Here's how the part is built. I have some questions about the finished solid (model axes, mm). A direction names the side the tool comes from. Round coordinates to 2 decimals unless told otherwise and drop trailing zeros. Loops run counter-clockwise (first coordinate to the right, second up) from the corner with the lowest first, then second, coordinate; pieces in that order, holes last. Notation, with made-up numbers: (-12.5, -33) - (4.5, -33) arc R16 ccw to (4.5, -14) - close; hole circle Ø11 at (-29, 0.25). An arc over 180 degrees is marked (long way). Answer as a JSON object with one key per item and string values. Group by question number.
1) If I drill on line 1 along Z through (x, y) = (0, -3.2); line 2 along Z through (x, y) = (0, -1.25), over which ranges is the centre line in solid material (lowest first)? Write a range as [from, to].
2) Will these pins go through, and if not, where does the flat tip stop? P1, Ø3, axis at y = 2.5, z = 7.5, coming from the -X side; P2, Ø2, axis at x = 4.5, y = 2.5, coming from the +Z side.
3) I want a section at C-C, the plane y = -1.25. Please give me the cut outline in (x, z), then the cut area to 3 significant figures.
4) I want a section at B-B, the plane x = -15. Please give me the cut outline in (y, z), then the cut area to 3 significant figures.
5) Which directions (+Z, -Z, +X, -X, +Y, -Y) give clear straight access to the entire face, cutting with the end or side of a thin tool? Please do faces 1 (the face through (20.03, 3.01, -6.31)), 2 (the face through (-14, -3.5, -21)), 3 (the face through (-5.7, -2.5, -20.5)).
6) I want a section at A-A, the plane z = 0. Please give me the cut outline in (x, y), then the cut area to 3 significant figures.
7) If we mould it in two halves opening along Z, with no side actions, what happens to faces 4 (the face through (-20.633, 0.049, 15.821)), 5 (the face through (-4.336, -0.049, 19.524)), 6 (the face through (-14, 3.5, -21))? For each: pulls with the +Z half, pulls with the -Z half, needs draft (parallel to the pull), parting line crosses it, or undercut.
from build123d import *

# Parameters (mm, degrees)
CROQUIS1_R              = 26
CROQUIS1_R_2            = 20
SALIENTE_EXTRUIR1_DEPTH = 3.5
CROQUIS2_R              = 25
CROQUIS2_R_2            = 21
CORTAR_EXTRUIR1_DEPTH   = 1


with BuildPart() as part:
    # Croquis1 → Saliente-Extruir1 (new body, symmetric)
    with BuildSketch(Plane(origin=(0, 0, 0), x_dir=(1, 0, 0), z_dir=(0, 1, 0))):
        Circle(CROQUIS1_R)
        Circle(CROQUIS1_R_2, mode=Mode.SUBTRACT)
    extrude(amount=SALIENTE_EXTRUIR1_DEPTH, both=True)

    # Croquis2 → Cortar-Extruir1 (cut)
    with BuildSketch(Plane(origin=(0, 3.5, 0), x_dir=(1, 0, 0), z_dir=(0, 1, 0))):
        Circle(CROQUIS2_R)
        Circle(CROQUIS2_R_2, mode=Mode.SUBTRACT)
    cortar_extruir1 = extrude(amount=-CORTAR_EXTRUIR1_DEPTH, mode=Mode.SUBTRACT)

    # Simetría1: Cortar-Extruir1 across plane
    add(cortar_extruir1.mirror(Plane.ZX), mode=Mode.SUBTRACT)


solid = part.part
Outcome:
{
 "1": {"line 1": "[-26, -25], [-21, -20], [20, 21], [25, 26]", "line 2": "[-26, -20], [20, 26]"},
 "2": {"P1": "x = -25.3", "P2": "z = 25.76"},
 "3": {"outline": "circle Ø52 at (0, 0); hole circle Ø40 at (0, 0)", "area": "867 mm^2"},
 "4": {"outline": "(-3.5, -21.24) - (3.5, -21.24) - (3.5, -20) - (2.5, -20) - (2.5, -14.7) - (3.5, -14.7) - (3.5, -13.23) - (-3.5, -13.23) - (-3.5, -14.7) - (-2.5, -14.7) - (-2.5, -20) - (-3.5, -20) - close; (-3.5, 13.23) - (3.5, 13.23) - (3.5, 14.7) - (2.5, 14.7) - (2.5, 20) - (3.5, 20) - (3.5, 21.24) - (-3.5, 21.24) - (-3.5, 20) - (-2.5, 20) - (-2.5, 14.7) - (-3.5, 14.7) - close", "area": "90.9 mm^2"},
 "5": {"face 1": "+Y", "face 2": "+Z, -Z, +X, -X, -Y", "face 3": "-Y"},
 "6": {"outline": "(-26, -3.5) - (-25, -3.5) - (-25, -2.5) - (-21, -2.5) - (-21, -3.5) - (-20, -3.5) - (-20, 3.5) - (-21, 3.5) - (-21, 2.5) - (-25, 2.5) - (-25, 3.5) - (-26, 3.5) - close; (20, -3.5) - (21, -3.5) - (21, -2.5) - (25, -2.5) - (25, -3.5) - (26, -3.5) - (26, 3.5) - (25, 3.5) - (25, 2.5) - (21, 2.5) - (21, 3.5) - (20, 3.5) - close", "area": "68.0 mm^2"},
 "7": {"face 4": "parting line crosses it", "face 5": "undercut", "face 6": "needs draft"}
}
